Verification items for the finished model (mm, model axes). A direction names the side the tool comes from. Coordinates: 2 decimals unless noted, no trailing zeros. Order: outer loops, then holes, each group sorted by start corner. A loop starts at its lowest first (then second) coordinate and runs counter-clockwise, first axis right, second up.
Q1. Draft check along Z on faces 4 (the flat face through (15.75, 2.39, 13.86)), 5 (the flat face through (7, -2.5, 25)). Enter one of: pulls with the +Z half, pulls with the -Z half, needs draft (parallel to the pull), parting line crosses it, or undercut.
Q2. Set-up check for faces 1 (the flat face through (-13.1, -8, 25)), 2 (the flat face through (-15.754, 2.37, 11.106)), 3 (the flat face through (7, 2.5, 25)): record each of +Z, -Z, +X, -X, +Y, -Y from which the full face is reachable in a straight line by a thin tool's end or side.
Q3. Cross-section at B-B, the plane z = 47. Record the boundary of the cut face in (x, y).
Q4. Thickness scan on line 1 (Z direction, x = 18.75, y = 0); line 2 (X direction, y = -11.5, z = 14); line 3 (Y direction, x = -11, z = 6). Record the ranges inside material, lowest first.
Q5. Depth check by flat-ended pin: P1, Ø4.5, axis at y = 4, z = 37.5, coming from the +X side; P2, Ø5, axis at x = 16, z = 6, coming from the +Y side; P3, Ø4.5, axis at y = -8, z = 25.5, coming from the +X side. Enter the tip coordinate at first touch or a pass-through.
Q6. Cross-section at A-A, the plane x = 0. Record the boundary of the cut face in (y, z).
Q7. Cross-section at C-C, the plane x = 8. Count the separate pieces of the cut face and the enclosed holes in it, and give its area (3 significant figures).
from build123d import *

# Parameters (mm, degrees)
SKETCH_1_R           = 21
EXTRUDE_1_DEPTH      = 50
FILLET_1_R           = 1
FILLET_2_R           = 1
SKETCH_2_R           = 2
CUT_EXTRUDE_1_DEPTH  = 43
CUT_EXTRUDE_START    = -5
CUT_EXTRUDE_2_DEPTH  = 2.4
CUT_EXTRUDE_9_DEPTH  = 51
SKETCH_6_W           = 2.4
SKETCH_6_H           = 5.5
CUT_EXTRUDE_10_DEPTH = 21
CUT_EXTRUDE_START_2  = -21
SKETCH_6_5_W         = 2.4
SKETCH_6_5_H         = 5.5
CUT_EXTRUDE_11_DEPTH = 21


with BuildPart() as part:
    # Эскиз1 → Бобышка-Вытянуть1 (new body)
    with BuildSketch(Plane.XY):
        Circle(SKETCH_1_R)
    extrude(amount=EXTRUDE_1_DEPTH)

    # Скругление1
    fillet_1_edges = [part.edges().sort_by_distance(p)[0] for p in [
        (-21, 0, 50),
    ]]
    fillet(fillet_1_edges, radius=FILLET_1_R)

    # Скругление2
    fillet_2_edges = [part.edges().sort_by_distance(p)[0] for p in [
        (-21, 0, 0),
    ]]
    fillet(fillet_2_edges, radius=FILLET_2_R)

    # Эскиз2 → Вырез-Вытянуть1 (cut, through all)
    with BuildSketch(Plane(origin=(21, 0, 0), x_dir=(0, 0, -1), z_dir=(1, 0, 0))):
        with Locations((-37.5, 0)):
            Circle(SKETCH_2_R)
        with Locations((-25, 0)):
            Circle(SKETCH_2_R)
        with Locations((-12.5, 0)):
            Circle(SKETCH_2_R)
    extrude(amount=-CUT_EXTRUDE_1_DEPTH, mode=Mode.SUBTRACT)

    # Эскиз3 → Вырез-Вытянуть2 (cut)
    with BuildSketch(Plane(origin=(21, 0, 0), x_dir=(0, 0, -1), z_dir=(1, 0, 0)).offset(CUT_EXTRUDE_START)):
        Polygon((-25, 3.175426481), (-27.75, 1.58771324), (-27.75, -1.58771324), (-25, -3.175426481), (-22.25, -1.58771324), (-22.25, 1.58771324), align=None)
        Polygon((-37.5, 3.175426481), (-40.25, 1.58771324), (-40.25, -1.58771324), (-37.5, -3.175426481), (-34.75, -1.58771324), (-34.75, 1.58771324), align=None)
        Polygon((-12.5, 3.175426481), (-15.25, 1.58771324), (-15.25, -1.58771324), (-12.5, -3.175426481), (-9.75, -1.58771324), (-9.75, 1.58771324), align=None)
    cut_extrude_2 = extrude(amount=-CUT_EXTRUDE_2_DEPTH, mode=Mode.SUBTRACT)

    # Зеркальное отражение1: Вырез-Вытянуть2 across plane
    add(cut_extrude_2.mirror(Plane(origin=(0, 0, 0), x_dir=(0, 0, 1), z_dir=(1, 0, 0))), mode=Mode.SUBTRACT)

    # Эскиз4 → Вырез-Вытянуть9 (cut, through all)
    with BuildSketch(Plane.XY.offset(50)):
        with BuildLine():
            Line((-2, 2.5), (-2, 12.338962679))
            ThreePointArc((-2, 12.338962679), (-8.657294344, 9.016720836), (-12.247448714, 2.5))
            Line((-12.247448714, 2.5), (-2, 2.5))
        make_face()
        with BuildLine():
            Line((2, 12.338962679), (2, 2.5))
            Line((2, 2.5), (12.247448714, 2.5))
            ThreePointArc((12.247448714, 2.5), (8.657294344, 9.016720836), (2, 12.338962679))
        make_face()
        with BuildLine():
            ThreePointArc((2, -12.338962679), (8.657294344, -9.016720836), (12.247448714, -2.5))
            Line((12.247448714, -2.5), (2, -2.5))
            Line((2, -2.5), (2, -12.338962679))
        make_face()
        with BuildLine():
            Line((-2, -2.5), (-12.247448714, -2.5))
            ThreePointArc((-12.247448714, -2.5), (-8.657294344, -9.016720836), (-2, -12.338962679))
            Line((-2, -12.338962679), (-2, -2.5))
        make_face()
    extrude(amount=-CUT_EXTRUDE_9_DEPTH, mode=Mode.SUBTRACT)

    # Эскиз6 → Вырез-Вытянуть10 (cut)
    with BuildSketch(Plane(origin=(0, 21, 0), x_dir=(1, 0, 0), z_dir=(0, 1, 0))):
        with Locations((14.3, -37.5)):
            Rectangle(SKETCH_6_W, SKETCH_6_H)
        with Locations((14.3, -12.5)):
            Rectangle(SKETCH_6_W, SKETCH_6_H)
    cut_extrude_10 = extrude(amount=-CUT_EXTRUDE_10_DEPTH, mode=Mode.SUBTRACT)

    # Эскиз6<5> → Вырез-Вытянуть11 (cut)
    with BuildSketch(Plane(origin=(0, 21, 0), x_dir=(1, 0, 0), z_dir=(0, 1, 0)).offset(CUT_EXTRUDE_START_2)):
        with Locations((14.3, -25)):
            Rectangle(SKETCH_6_5_W, SKETCH_6_5_H)
    cut_extrude_11 = extrude(amount=-CUT_EXTRUDE_11_DEPTH, mode=Mode.SUBTRACT)

    # Зеркальное отражение2: Вырез-Вытянуть10, Вырез-Вытянуть11 across plane
    add(cut_extrude_10.mirror(Plane(origin=(0, 0, 0), x_dir=(0, 0, 1), z_dir=(1, 0, 0))), mode=Mode.SUBTRACT)
    add(cut_extrude_11.mirror(Plane(origin=(0, 0, 0), x_dir=(0, 0, 1), z_dir=(1, 0, 0))), mode=Mode.SUBTRACT)


solid = part.part
Check values:
1. face 4: undercut
1. face 5: needs draft
2. face 1: -Y
2. face 2: none
2. face 3: +Z, -Z
3. outline: circle Ø42 at (0, 0); hole (-12.25, -2.5) arc R12.5 ccw to (-2, -12.34) - (-2, -2.5) - close; hole (-12.25, 2.5) - (-2, 2.5) - (-2, 12.34) arc R12.5 ccw to start; hole (2, -12.34) arc R12.5 ccw to (12.25, -2.5) - (2, -2.5) - close; hole (2, 2.5) - (12.25, 2.5) arc R12.5 ccw to (2, 12.34) - close
4. line 1: z = 0 to 10.5, 14.5 to 23, 27 to 35.5, 39.5 to 50
4. line 2: x = -17.57 to -4.9, -2 to 2, 4.9 to 17.57
4. line 3: y = -17.89 to -5.94, -2.5 to 2.5, 5.94 to 17.89
5. P1: stops at x = 20.92
5. P2: stops at y = 16.09
5. P3: stops at x = 20.2
6. outline: (-21, 1) arc R1 ccw to (-20, 0) - (20, 0) arc R1 ccw to (21, 1) - (21, 49) arc R1 ccw to (20, 50) - (-20, 50) arc R1 ccw to (-21, 49) - close; hole circle Ø4 at (0, 12.5); hole circle Ø4 at (0, 25); hole circle Ø4 at (0, 37.5)
7. separate pieces: 3
7. enclosed holes: 3
7. area: 1,190 mm2
